CAD build for the part. Positions are in the model's coordinates, mm. A direction names the side the tool comes from. Give positions to 0.01 mm unless a question says otherwise; leave off trailing zeros. Order: outer loops, then holes, each group sorted by start corner. A loop starts at its lowest first (then second) coordinate and runs counter-clockwise, first axis right, second up. Notation, with made-up numbers: (81, 45.5) -> (118, 45.5) arc R18 cw to (118, 53.5) -> close; hole circle Ø11 at (4.5, 56). An arc over 180 degrees is marked (long way). Use one line per item in the form item = value. Start each with the question number.
1) Tool access for faces 1 (the face through (0, 1, 0)), 2 (the face through (-10, -1, 986)): list every direction of +Z, -Z, +X, -X, +Y, -Y with a clear straight run to the whole face (end or side of a thin tool).
2) Cut at B-B, the plane y = 30.5. Give the cut face in (x, z).
3) Drop flat-ended pins along their axis: P1, Ø3, axis at y = -3.5, z = 1540.5, coming from the -X side; P2, Ø4, axis at y = 27.5, z = 1383.5, coming from the +X side. Give the stop position or say it passes through.
4) Mould opens along Y. For faces 3 (the face through (0, 70, 986)), 4 (the face through (0, -70, 986)), 5 (the face through (10, -1, 986)) say: pulls with the +Y half, pulls with the -Y half, needs draft (parallel to the pull), parting line crosses it, or undercut.
5) Cut at A-A, the plane z = 705. Give the cut face in (x, y).
6) Probe line 1 (Y direction, x = -27, z = 1599); line 2 (X direction, y = 19, z = 505). List the from-to ranges inside material, lowest first.
Autodesk Inventor part; units mm, degrees
ref_plane "YZ Plane" through (0, 0, 0) normal (1, 0, 0) x (0, 1, 0)
ref_plane "XZ Plane" through (0, 0, 0) normal (0, 1, 0) x (-1, 0, 0)
ref_plane "XY Plane" through (0, 0, 0) normal (0, 0, 1) x (1, 0, 0)
sketch "Sketch1" plane through (0, 0, 0) normal (0, 0, 1) x (1, 0, 0)
  line L0 (10, 0) -> (10, 50)
  line L1 (10, 50) -> (30, 50)
  line L2 (30, 50) -> (30, 70)
  line L3 (30, 70) -> (0, 70)
  line L4 (10, 0) -> (10, -50)
  line L5 (10, -50) -> (30, -50)
  line L6 (30, -50) -> (30, -70)
  line L7 (30, -70) -> (0, -70)
  line L8 (-10, 0) -> (-10, 50)
  line L9 (-10, 50) -> (-30, 50)
  line L10 (-30, 50) -> (-30, 70)
  line L11 (-30, 70) -> (0, 70)
  line L12 (-10, 0) -> (-10, -50)
  line L13 (-10, -50) -> (-30, -50)
  line L14 (-30, -50) -> (-30, -70)
  line L15 (-30, -70) -> (0, -70)
  point P0 (0, 0)
  dimension "d4" = 50
  dimension "d5" = 20
  dimension "d6" = 20
extrude "Extrusion1" add sketch "Sketch1" along normal blind 2000
properties part number "A Console beam" material "Steel, Cast"
Result:
q1.face_1 = -Z, +X, -X, +Y, -Y
q1.face_2 = +Z, -Z, -X
q2.outline = (-10, 0) -> (10, 0) -> (10, 2000) -> (-10, 2000) -> close
q3.P1 = -10
q3.P2 = 10
q4.face_3 = pulls with the +Y half
q4.face_4 = pulls with the -Y half
q4.face_5 = undercut
q5.outline = (-30, -70) -> (30, -70) -> (30, -50) -> (10, -50) -> (10, 50) -> (30, 50) -> (30, 70) -> (-30, 70) -> (-30, 50) -> (-10, 50) -> (-10, -50) -> (-30, -50) -> close
q6.line_1 = -70 to -50, 50 to 70
q6.line_2 = -10 to 10
